The figure shows three views and two pictorial views of one solid part (mm, origin at its lowest corner). Answer the questions. Coordinates: 2 decimals unless noted, no trailing zeros. Order: outer loops, then holes, each group sorted by start corner. A loop starts at its lowest first (then second) coordinate and runs counter-clockwise, first axis right, second up. Notation, with made-up numbers: (0, -31) -> (16, -31) arc R21 cw to (16, -17) -> close; hole circle Ø8 at (9.25, -31.75). An arc over 180 degrees is marked (long way). Write item = value, one per line.
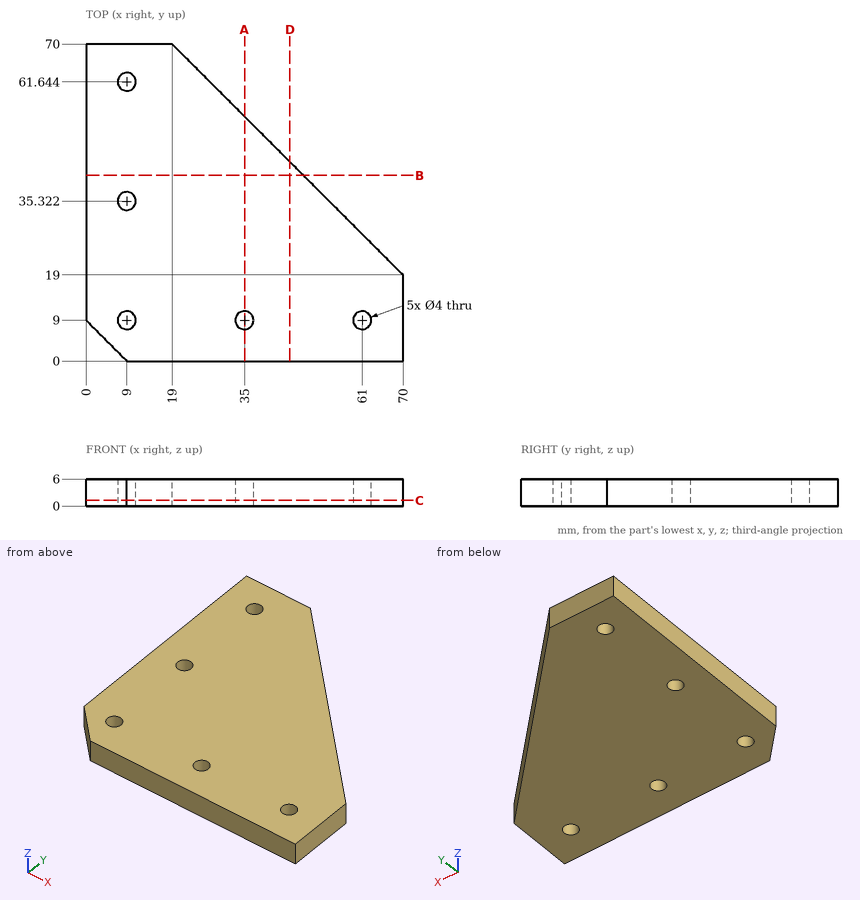
Q1. Section D-D, the plane x = 45 is taken. Give the vertices of the cut face in (y, z), plus the area to 3 significant figures.
The answers:
outline = (0, 0) -> (44, 0) -> (44, 6) -> (0, 6) -> close
area = 264 mm2
Q2. Section A-A, the plane x = 35 is taken. Give the vertices of the cut face in (y, z), plus the area to 3 significant figures.
The answers:
outline = (0, 0) -> (7, 0) -> (7, 6) -> (0, 6) -> close; (11, 0) -> (54, 0) -> (54, 6) -> (11, 6) -> close
area = 300 mm2
Q3. This flat-tipped pin is pushed along its axis until it touches: pin 1 Ø4 at (x, y) = (42, 11.5) entering from -Z. Where does it stop, or does it pass through?
The answers:
pin_1 = 0
Q4. Section B-B, the plane y = 41 is taken. Give the vertices of the cut face in (x, z).
The answers:
outline = (0, 0) -> (48, 0) -> (48, 6) -> (0, 6) -> close
Q5. Section C-C, the plane z = 1.3 is taken. Give the vertices of the cut face in (x, y).
The answers:
outline = (0, 9) -> (9, 0) -> (70, 0) -> (70, 19) -> (19, 70) -> (0, 70) -> close; hole circle Ø4 at (9, 9); hole circle Ø4 at (9, 35.32); hole circle Ø4 at (9, 61.64); hole circle Ø4 at (35, 9); hole circle Ø4 at (61, 9)
Q6. Find the intervals of material crossed by line 1 along Y through (x, z) = (9, 1.45); line 2 along Y through (x, z) = (33.5, 0.85); line 3 along X through (y, z) = (8.5, 0.4), in increasing order.
The answers:
line_1 = 0 to 7, 11 to 33.32, 37.32 to 59.64, 63.64 to 70
line_2 = 0 to 7.68, 10.32 to 55.5
line_3 = 0.5 to 7.06, 10.94 to 33.06, 36.94 to 59.06, 62.94 to 70
